Design review of the part built by this model. Coordinates are the model's own, in mm. A direction names the side the tool comes from. Coordinates: 2 decimals unless noted, no trailing zeros.
from build123d import *

# Parameters (mm, degrees)
SKETCH2_R           = 7.5
SKETCH2_R_2         = 5.5
BOSS_EXTRUDE1_DEPTH = 2.5


with BuildPart() as part:
    # Sketch1 → Revolve1 (revolve)
    with BuildSketch(Plane.XY, mode=Mode.PRIVATE) as revolve1_sk:
        Polygon((-0.855365474, 120), (-10, 120), (-10, 140), (-15, 140), (-15, 115), (-6, 106), (-6, 30), (-60, 10), (-60, 0), (0, 0), align=None)
    revolve(revolve1_sk.sketch.rotate(Axis((-0.855365474, 120, 0), (0.0071278645418364215, -0.9999745964508665, 0)), 180), axis=Axis((-0.855365474, 120, 0), (0.0071278645418364215, -0.9999745964508665, 0)))

    # Sketch2 → Boss-Extrude1 (add, symmetric)
    with BuildSketch(Plane.XY):
        with Locations((30.571729314, 27.591749237)):
            Circle(SKETCH2_R)
        with Locations((30.571729314, 27.591749237)):
            Circle(SKETCH2_R_2, mode=Mode.SUBTRACT)
    extrude(amount=BOSS_EXTRUDE1_DEPTH, both=True)


solid = part.part
Q1. For line 1 (Y direction, x = -31.5, z = 46); line 2 (Y direction, x = -16.5, z = -35); line 3 (Z direction, x = 25.5, y = 8), list the stretches that pass through material, from the lowest coordinate up.
Q2. The part is to be moulded in two halves that separate along X. For faces 5 (the cylindrical face through (25.077, 27.834, -0.035)), 6 (the conical face through (-13.037, 5.265, -58.537)), 7 (the flat face through (33, 33, -2.5)), say which applies: pulls with the +X half, pulls with the -X half, needs draft (parallel to the pull), parting line crosses it, or undercut.
Q3. Clearance check with flat-ended pins moving along their axes: pin 1 Ø10 at (x, z) = (-26.5, -27.5) entering from +Y; pin 2 Ø12 at (x, y) = (-19.5, 113.5) entering from -Z; pin 3 Ø1.5 at (y, z) = (77.5, 2.5) entering from -X; pin 4 Ø4.5 at (x, y) = (28, 26) entering from -Z. State where each tip first meets the part, or that it passes through.
Q4. Machinability: for faces 1 (the flat face through (33, 33, 2.5)), 2 (the conical face through (-2.312, 0.004, -1.773)), 3 (the conical face through (7.725, 130.266, 2.725)), 4 (the conical face through (6.67, 127.48, 11.88)), which of the approach directions +Z, -Z, +X, -X, +Y, -Y give a long, thin tool a straight path to every point of the face, cutting with its end or side? Answer none if there is none.
Entries:
1. line 1: y = 0.17 to 11.73
1. line 2: y = 0.16 to 18.02
1. line 3: z = -54.23 to 54.23
2. face 5: undercut
2. face 6: parting line crosses it
2. face 7: needs draft
3. pin 1: stops at y = 19.99
3. pin 2: stops at z = -5.95
3. pin 3: stops at x = -5.71
3. pin 4: passes through
4. face 1: +Z, +X, +Y
4. face 2: +X, -Y
4. face 3: none
4. face 4: +Y
